```python
from build123d import *

# Parameters (mm, degrees)
SKETCH_2_R          = 4
CUT_EXTRUDE_1_DEPTH = 10
FILLET_1_R          = 2


with BuildPart() as part:
    # Эскиз1 → Повернуть1 (revolve)
    with BuildSketch(Plane.XY, mode=Mode.PRIVATE) as revolve_1_sk:
        Polygon((-26.283026585, 8), (-26.283026585, 0), (-20.283026585, 0), (-20.283026585, 8), (-22.783026585, 8), (-22.783026585, 6), (-23.783026585, 6), (-23.783026585, 8), align=None)
    revolve(revolve_1_sk.sketch.rotate(Axis((-31.114528332, 0, 0), (1, 0, 0)), 90), axis=Axis((-31.114528332, 0, 0), (1, 0, 0)))

    # Эскиз2 → Вырез-Вытянуть1 (cut)
    with BuildSketch(Plane(origin=(-20.283026585, 0, 0), x_dir=(0, 0, -1), z_dir=(1, 0, 0))):
        Circle(SKETCH_2_R)
    extrude(amount=-CUT_EXTRUDE_1_DEPTH, mode=Mode.SUBTRACT)

    # Скругление1
    fillet_1_edges = [part.edges().sort_by_distance(p)[0] for p in [
        (-26.283026585, 0, -8),
        (-20.283026585, 0, -8),
    ]]
    fillet(fillet_1_edges, radius=FILLET_1_R)


solid = part.part
```
Work out the finished part from the listing and answer in its coordinate system (mm). A direction names the side the tool comes from. Round coordinates to 2 decimals unless told otherwise and drop trailing zeros. Write each loop counter-clockwise with the first axis right and the second up, starting at its lowest first coordinate (ties: lowest second). Pieces come first, ordered by that corner, then holes.
1) Which of the six approach directions +Z, -Z, +X, -X, +Y, -Y give full straight-line access (tool end or side, diameter ignored) to faces 1 (the face through (-24.04, 7.81, -1.73)), 2 (the face through (-22.783, -6, -2))?
2) Consider probe 1 along Y at (x, z) = (-22.1, 0); probe 2 along Y at (x, z) = (-25.25, -3.25); probe 3 along Z at (x, y) = (-25.6, 1.75). Determine where each line is inside the solid, lowest interval first.
3) A cutting plane is placed at C-C on x = -25.2. Determine the outline of the cut face in (y, z), and give its area (3 significant figures).
4) Flat-ended cylindrical pins translate along their axes: P1, Ø3, axis at x = -25, y = -5, coming from the +Z side; P2, Ø1, axis at x = -23, z = -4.5, coming from the +Y side. Find the tip coordinate at first contact, or state that the pin passes through.
5) A cutting plane is placed at D-D on x = -20.9. Determine the outline of the cut face in (y, z).
6) A cutting plane is placed at A-A on y = 0. Determine the outline of the cut face in (x, z).
7) Determine the mould class of faces 3 (the face through (-20.283, 3.92, 1.42)), 4 (the face through (-22.54, 7.81, -1.73)), 5 (the face through (-23.241, -3.905, 0.867)) for opening direction Y: pulls with the +Y half, pulls with the -Y half, needs draft (parallel to the pull), parting line crosses it, or undercut.
Entries:
1. face 1: +X, -X
1. face 2: none
2. probe 1: y = -7.99 to -4, 4 to 7.99
2. probe 2: y = -7.04 to -2.33, 2.33 to 7.04
2. probe 3: z = -7.3 to -3.6, 3.6 to 7.3
3. outline: circle Ø15.55 at (0, 0); hole circle Ø8 at (0, 0)
3. area: 140 mm2
4. P1: stops at z = 7.14
4. P2: stops at y = 6.9
5. outline: circle Ø14.89 at (0, 0); hole circle Ø8 at (0, 0)
6. outline: (-26.28, -6) arc R2 ccw to (-24.28, -8) - (-23.78, -8) - (-23.78, -6) - (-22.78, -6) - (-22.78, -8) - (-22.28, -8) arc R2 ccw to (-20.28, -6) - (-20.28, -4) - (-26.28, -4) - close; (-26.28, 4) - (-20.28, 4) - (-20.28, 6) arc R2 ccw to (-22.28, 8) - (-22.78, 8) - (-22.78, 6) - (-23.78, 6) - (-23.78, 8) - (-24.28, 8) arc R2 ccw to (-26.28, 6) - close
7. face 3: needs draft
7. face 4: parting line crosses it
7. face 5: undercut
